For this review, use the dimensioned drawing (mm, ordinates from the lowest corner) and the shaded views. Round coordinates to 2 decimals unless told otherwise and drop trailing zeros. Write each loop counter-clockwise with the first axis right and the second up, starting at its lowest first coordinate (ties: lowest second). Pieces come first, ordered by that corner, then holes.
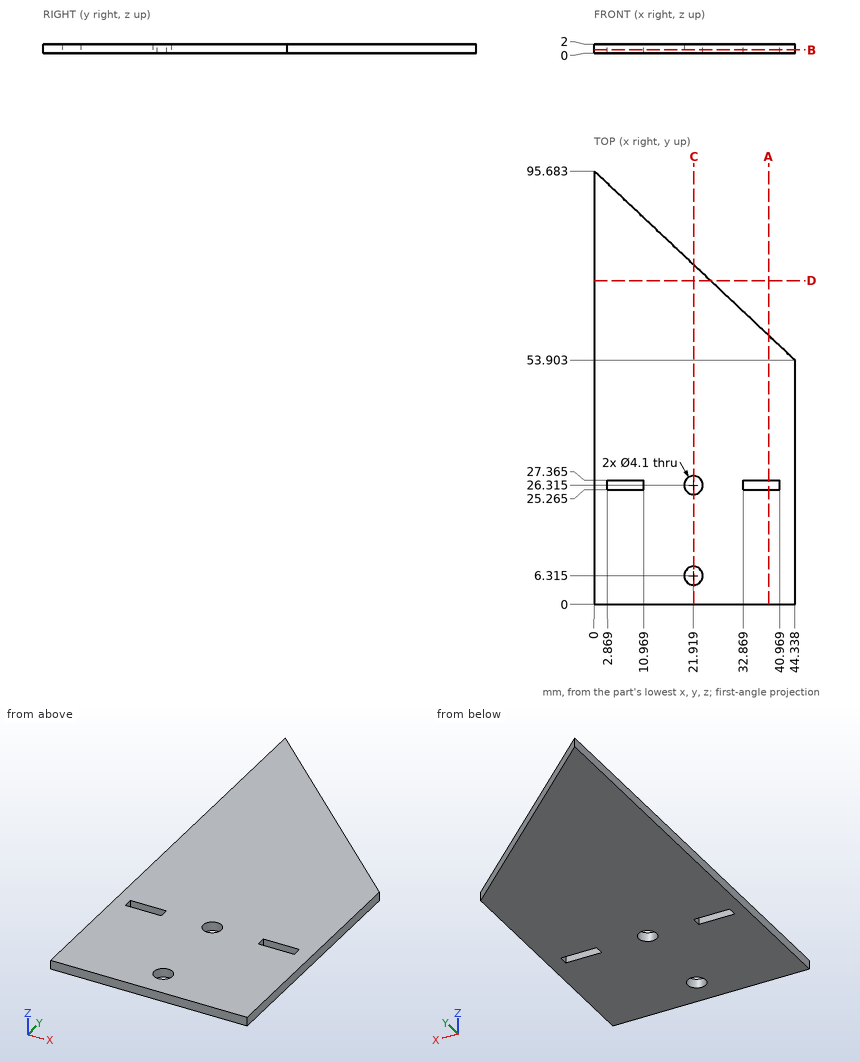
1) Add section C-C on x = 22. State the section outline as (y, z) points.
2) Add section D-D on y = 71.5. State the section outline as (x, z) points.
3) Add section A-A on x = 38.5. State the section outline as (y, z) points (1 decimal).
4) For P1, Ø1, axis at x = 6.5, z = 1.5, coming from the +Y side; P2, Ø0.6, axis at x = 38.5, z = 1, coming from the +Y side (1 decimal); P3, Ø2.5, axis at x = 21.92, y = 26.31, coming from the -Z side, all flat-tipped, find the tip position at first contact; note any pin that passes through.
5) For line 1 along X through (y, z) = (5.5, 1.8); line 2 along Y through (x, z) = (19.5, 0.5); line 3 along Y through (x, z) = (24, 0.45) (1 decimal), list the stretches that pass through material, from the lowest coordinate up.
6) Add section B-B on z = 0.7. Count the separate pieces of the cut face and the enclosed holes in it, and give its area (3 significant figures).
Computed:
1. outline: (0, 0) - (4.27, 0) - (4.27, 2) - (0, 2) - close; (8.36, 0) - (24.27, 0) - (24.27, 2) - (8.36, 2) - close; (28.36, 0) - (74.95, 0) - (74.95, 2) - (28.36, 2) - close
2. outline: (0, 0) - (25.66, 0) - (25.66, 2) - (0, 2) - close
3. outline: (0, 0) - (25.3, 0) - (25.3, 2) - (0, 2) - close; (27.4, 0) - (59.4, 0) - (59.4, 2) - (27.4, 2) - close
4. P1: stops at y = 90.03
4. P2: stops at y = 59.7
4. P3: passes through
5. line 1: x = 0 to 20.04, 23.8 to 44.34
5. line 2: y = 0 to 77.31
5. line 3: y = 0 to 73.1
6. separate pieces: 1
6. enclosed holes: 4
6. area: 3,260 mm2
